Source: three-view drawing plus pictorial views. Frame: mm from the lowest corner of the part. A direction names the side the tool comes from. Coordinates: 2 decimals unless noted, no trailing zeros. Order: outer loops, then holes, each group sorted by start corner. A loop starts at its lowest first (then second) coordinate and runs counter-clockwise, first axis right, second up. Notation, with made-up numbers: M 20.5,75.25 L 77.5,75.25 A6 cw 77.5,85.25 Z; hole C 88.5,82.25 d8. An arc over 180 degrees is marked long. One line per question, with ' | ' between items.
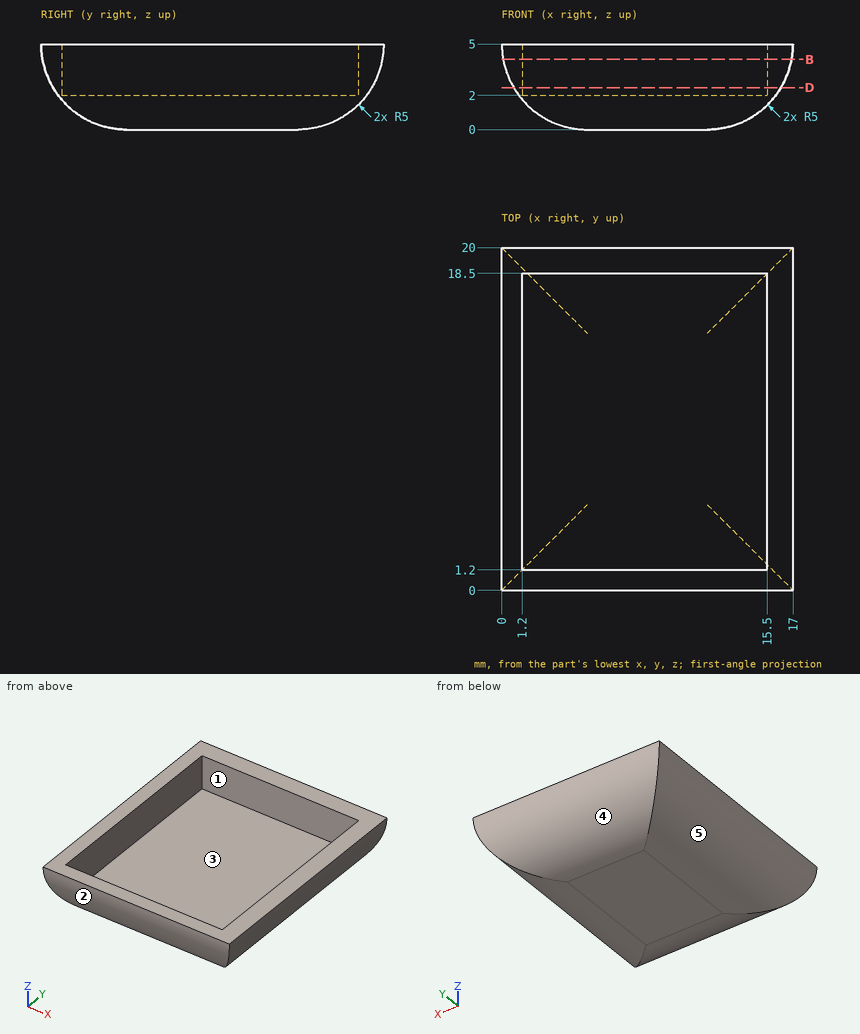
1. Section D-D, the plane z = 2.45. Output: boundary loops of the cut face in (x, y), and give its area (3 significant figures).
Response values:
outline: M 0.7,0.7 L 16.3,0.7 L 16.3,19.3 L 0.7,19.3 Z; hole M 1.2,1.2 L 15.5,1.2 L 15.5,18.5 L 1.2,18.5 Z | area: 42.8 mm^2
2. Draft query along Y for the marked faces 3, 4 and 5. Return one class per face: pulls with the +Y half, pulls with the -Y half, needs draft (parallel to the pull), parting line crosses it, or undercut.
Response values:
face 3: undercut | face 4: pulls with the +Y half | face 5: needs draft
3. Pin query (flat end, axial travel): P1, Ø2.5, axis at y = 7, z = 3, coming from the -X side; P2, Ø0.9, axis at x = 7, z = 3, coming from the +Y side; P3, Ø0.9, axis at y = 7, z = 3.5, coming from the +X side. Return the tip coordinate at first contact, or that it passes through.
Response values:
P1: stops at x = 0.06 | P2: stops at y = 19.75 | P3: stops at x = 16.89
4. Section B-B, the plane z = 4.1. Output: boundary loops of the cut face in (x, y).
Response values:
outline: M 0.08,0.08 L 16.92,0.08 L 16.92,19.92 L 0.08,19.92 Z; hole M 1.2,1.2 L 15.5,1.2 L 15.5,18.5 L 1.2,18.5 Z
5. Access query for the marked faces 1 and 2. Directions: +Z, -Z, +X, -X, +Y, -Y. A direction counts if a zero-diameter tool reaches every point of the face in a straight line with its end or side. Return the directions, or none.
Response values:
face 1: +Z | face 2: -Z, +X, -X, -Y
6. Material intervals for line 1 (Z direction, x = 15.25, y = 8.25); line 2 (Z direction, x = 7.25, y = 14.5); line 3 (Y direction, x = 6, z = 4.7), sorted ascending. Write a range as [from, to].
Response values:
line 1: z = [1.2, 2] | line 2: z = [0, 2] | line 3: y = [0.01, 1.2], [18.5, 19.99]
